```python
from build123d import *
from OCP.BRepFilletAPI import BRepFilletAPI_MakeChamfer

# Parameters (mm, degrees)
SKETCH_1_W          = 50
SKETCH_1_H          = 22
EXTRUDE_1_DEPTH     = 10
CUT_EXTRUDE_1_DEPTH = 2
CUT_EXTRUDE_2_DEPTH = 1
CHAMFER_1_SIZE      = 1
CHAMFER_2_SIZE      = 1
CHAMFER_2_SIZE_2    = 1.732050808
FILLET_1_R          = 1


with BuildPart() as part:
    # 草图1 → 凸台-拉伸1 (new body)
    with BuildSketch(Plane(origin=(0, 0, 0), x_dir=(1, 0, 0), z_dir=(0, 1, 0))):
        with Locations((25, 11)):
            Rectangle(SKETCH_1_W, SKETCH_1_H)
        with BuildLine():
            Line((22, 6.5), (10, 6.5))
            ThreePointArc((10, 6.5), (5.5, 11), (10, 15.5))
            Line((10, 15.5), (22, 15.5))
            ThreePointArc((22, 15.5), (26.5, 11), (22, 6.5))
        make_face(mode=Mode.SUBTRACT)
    extrude(amount=EXTRUDE_1_DEPTH)

    # 草图2 → 切除-拉伸1 (cut)
    with BuildSketch(Plane.XZ):
        with BuildLine():
            Line((50, -6.5), (50, -15.5))
            Line((50, -15.5), (10, -15.5))
            ThreePointArc((10, -15.5), (5.5, -11), (10, -6.5))
            Line((10, -6.5), (50, -6.5))
        make_face()
    extrude(amount=-CUT_EXTRUDE_1_DEPTH, mode=Mode.SUBTRACT)

    # 草图3 → 切除-拉伸2 (cut)
    with BuildSketch(Plane.XZ):
        Polygon((0, -6.5), (5.5, -6.5), (5.5, 0), (14.5, 0), (14.5, -22), (5.5, -22), (5.5, -15.5), (0, -15.5), align=None)
    extrude(amount=-CUT_EXTRUDE_2_DEPTH, mode=Mode.SUBTRACT)

    # 倒角1
    chamfer_1_edges = [part.edges().sort_by_distance(p)[0] for p in [
        (0, 0, -18.75),
        (5.5, 0, -18.75),
        (5.5, 0, -3.25),
        (0, 0, -3.25),
    ]]
    chamfer(chamfer_1_edges, length=CHAMFER_1_SIZE - 0.0001)  # a hair under: the kernel refuses the full size

    # 倒角2
    chamfer_2_edges_1 = [part.edges().sort_by_distance(p)[0] for p in [
        (14.5, 0, -18.75),
    ]]
    chamfer_2_side_1 = [part.faces().sort_by_distance(p)[0] for p in [
        (14.5, 0.02, -18.75),
    ]]
    chamfer_2_edges_2 = [part.edges().sort_by_distance(p)[0] for p in [
        (14.5, 0, -3.25),
    ]]
    chamfer_2_side_2 = [part.faces().sort_by_distance(p)[0] for p in [
        (14.5, 0.02, -3.25),
    ]]
    chamfer_2 = BRepFilletAPI_MakeChamfer(part.part.solid().wrapped)
    for e in chamfer_2_edges_1:
        chamfer_2.Add(CHAMFER_2_SIZE - 0.0001, CHAMFER_2_SIZE_2 - 0.0001, e.wrapped, chamfer_2_side_1[0].wrapped)
    for e in chamfer_2_edges_2:
        chamfer_2.Add(CHAMFER_2_SIZE - 0.0001, CHAMFER_2_SIZE_2 - 0.0001, e.wrapped, chamfer_2_side_2[0].wrapped)
    add(Compound.cast(chamfer_2.Shape()), mode=Mode.REPLACE)  # a hair under: the kernel refuses the full size

    # 圆角1
    fillet_1_edges = [part.edges().sort_by_distance(p)[0] for p in [
        (25, 10, -22),
        (50, 10, -11),
        (25, 10, 0),
        (0, 10, -11),
        (50, 5, 0),
        (50, 5, -22),
        (0, 5.49995, -22),
        (0, 5.49995, 0),
        (50, 0, -18.75),
        (50, 0, -3.25),
    ]]
    fillet(fillet_1_edges, radius=FILLET_1_R)


solid = part.part
```
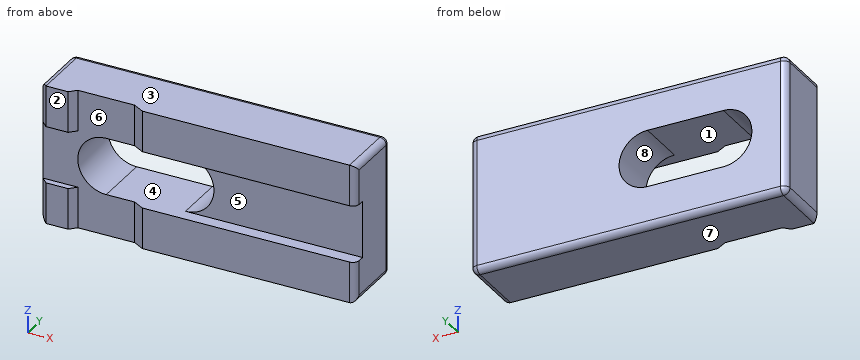
Geometry check sheet. Reference: the model listing, model coordinates, mm. Face numbers are marked on the shaded views. A direction names the side the tool comes from. Coordinates: 2 decimals unless noted, no trailing zeros. Write each loop counter-clockwise with the first axis right and the second up, starting at its lowest first coordinate (ties: lowest second). Pieces come first, ordered by that corner, then holes. Notation, with made-up numbers: M 13,8.25 L 22,8.25 A9 cw 22,20.25 Z; hole C 52,-35 d3. An arc over 180 degrees is marked long. Answer as a JSON object with one key per item and string values.
1. Section check C-C, the plane y = 5.5. Enter the section's corners in (x, z).
Answers below:
{"outline": "M 0,-21 A1 ccw 1,-22 L 49,-22 A1 ccw 50,-21 L 50,-1 A1 ccw 49,0 L 1,0 A1 ccw 0,-1 Z; hole M 10,-15.5 L 22,-15.5 A4.5 ccw 22,-6.5 L 10,-6.5 A4.5 ccw Z"}
2. Section check B-B, the plane x = 17.5. Enter the section's corners in (y, z).
Answers below:
{"outline": "M 0,-22 L 9,-22 A1 ccw 10,-21 L 10,-15.5 L 0,-15.5 Z; M 0,-6.5 L 10,-6.5 L 10,-1 A1 ccw 9,0 L 0,0 Z"}
3. Scan lines: L1, parallel to Z at x = 23, y = 1.75; L2, parallel to Y at x = 4.5, z = -7; L3, parallel to Y at x = 33, z = -14. Record each from-to range of solid material in increasing order.
Answers below:
{"L1": "z = -22 to -15.5, -6.5 to 0", "L2": "y = 1 to 10", "L3": "y = 2 to 10"}
4. Draft check along Z on the marked faces 1, 2, 3 and 4. Enter one of: released by +Z, released by -Z, zero draft, split by the parting line, or undercut.
Answers below:
{"face 1": "undercut", "face 2": "zero draft", "face 3": "released by +Z", "face 4": "undercut"}
5. Section check A-A, the plane z = -11. Enter the section's corners in (x, y), plus the area to 3 significant figures.
Answers below:
{"outline": "M 0,1 L 5.5,1 L 5.5,10 L 1,10 A1 ccw 0,9 Z; M 26.5,2 L 50,2 L 50,9 A1 ccw 49,10 L 26.5,10 Z", "area": "237 mm²"}
6. Tool access check on the marked faces 5, 6, 7 and 8. Record the directions out of +Z, -Z, +X, -X, +Y, -Y that give a thin tool (end or side, any length) a straight path to the whole face; none if there is none.
Answers below:
{"face 5": "+X, -Y", "face 6": "-Y", "face 7": "-Z, +X, -X, +Y, -Y", "face 8": "+Y, -Y"}
